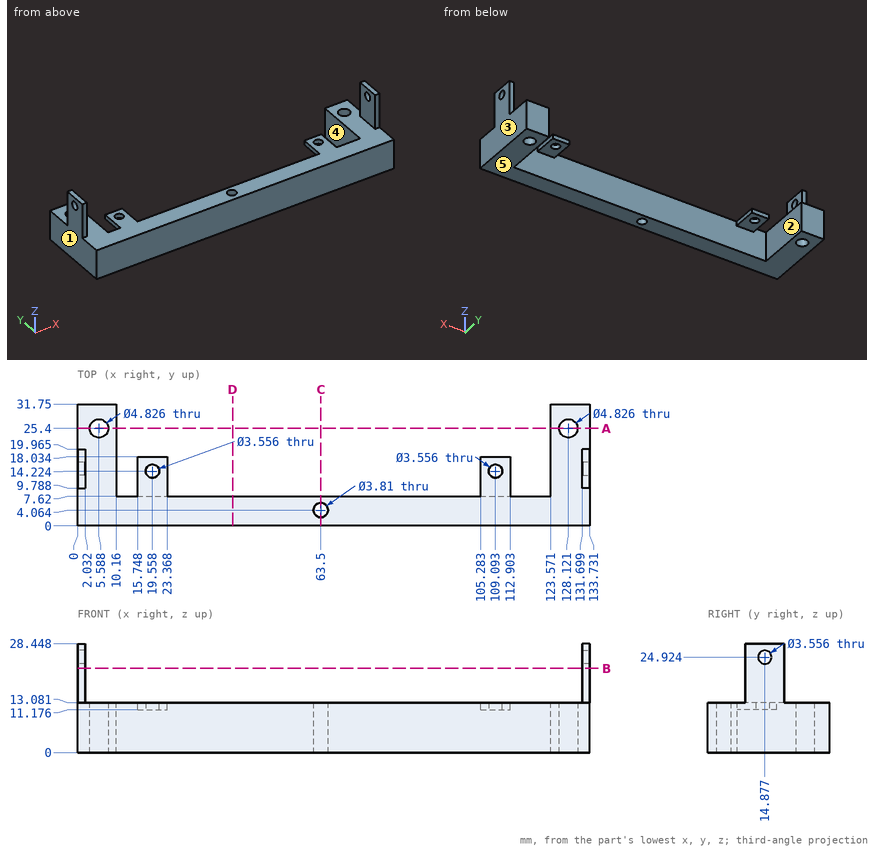
Study the drawing (mm; zero at the part's minimum x, y, z) and answer. A direction names the side the tool comes from. Round coordinates to 2 decimals unless told otherwise and drop trailing zeros. Order: outer loops, then holes, each group sorted by start corner. A loop starts at its lowest first (then second) coordinate and runs counter-clockwise, first axis right, second up. Notation, with made-up numbers: (64.25, -10) -> (81.25, -10) arc R17 cw to (81.25, 21) -> close; hole circle Ø5 at (-22.5, -30). An arc over 180 degrees is marked (long way). Answer as CSV lines item,"result". Start each with the question number.
(1) For a pull along X with two mould halves and no side action, classify the marked faces 3, 4 and 5 as +X half, -X half, draft (parallel to the pull), parting line (faces both ways), or undercut.
(2) The part is cut by section C-C (x = 63.5). Determine the outline of the cut face in (y, z).
(3) The part is cut by section D-D (x = 40.5). Determine the outline of the cut face in (y, z).
(4) Find the intervals of material crossed by probe 1 along X at (y, z) = (9, 5.5); probe 2 along X at (y, z) = (24.5, 4.75); probe 3 along X at (y, z) = (13.5, 21), in increasing order. Write a range as from..to.
(5) The part is cut by section B-B (z = 22). Determine the outline of the cut face in (x, y) (1 decimal).
(6) Flat-ended cylindrical pins translate along their axes: pin 1 Ø4 at (y, z) = (14.88, 24.92) entering from -X; pin 2 Ø1 at (x, z) = (1.5, 24) entering from -Y; pin 3 Ø6 at (x, y) = (108.5, 11) entering from -Z; pin 4 Ø1 at (x, z) = (132.5, 21.5) entering from +Y (1 decimal). Find the tip coordinate at first contact, or state that the pin passes through.
(7) The part is cut by section A-A (y = 25.4). Determine the outline of the cut face in (x, z) (1 decimal).
(8) A tool of negligible diameter and unlimited length cuts with its end or side. For the marked faces 1 and 2, from which of +Z, -Z, +X, -X, +Y, -Y can it reach the whole face along a straight path? Write none if from no direction.
Evaluation:
1,face 3,"+X half"
1,face 4,"undercut"
1,face 5,"draft"
2,outline,"(0, 0) -> (2.16, 0) -> (2.16, 13.08) -> (0, 13.08) -> close; (5.97, 0) -> (7.62, 0) -> (7.62, 13.08) -> (5.97, 13.08) -> close"
3,outline,"(0, 0) -> (7.62, 0) -> (7.62, 13.08) -> (0, 13.08) -> close"
4,probe 1,"0..10.16, 123.57..133.73"
4,probe 2,"0..3.35, 7.83..10.16, 123.57..125.88, 130.36..133.73"
4,probe 3,"0..2.03, 131.7..133.73"
5,outline,"(0, 9.8) -> (2, 9.8) -> (2, 20) -> (0, 20) -> close; (131.7, 9.8) -> (133.7, 9.8) -> (133.7, 20) -> (131.7, 20) -> close"
6,pin 1,"x = 0"
6,pin 2,"y = 9.79"
6,pin 3,"z = 11.18"
6,pin 4,"y = 20"
7,outline,"(0, 0) -> (3.2, 0) -> (3.2, 13.1) -> (0, 13.1) -> close; (8, 0) -> (10.2, 0) -> (10.2, 13.1) -> (8, 13.1) -> close; (123.6, 0) -> (125.7, 0) -> (125.7, 13.1) -> (123.6, 13.1) -> close; (130.5, 0) -> (133.7, 0) -> (133.7, 13.1) -> (130.5, 13.1) -> close"
8,face 1,"+Z, -Z, -X, +Y, -Y"
8,face 2,"+Z, -Z, +Y"
